from build123d import *

# Parameters (mm, degrees)
F0_W     = 120
F0_H     = 240
F0_R     = 2
F0_R_2   = 50.25
F1_DEPTH = 15
F0_R_3   = 1.75
F2_DEPTH = 12
F0_R_4   = 2.5
F0_R_5   = 51.75
F3_DEPTH = 10.5


with BuildPart() as f1:
    # F0 (on Right) → F1 (new body)
    with BuildSketch(Plane.YZ):
        with Locations((0, -1.592548)):
            Rectangle(F0_W, F0_H)
        with Locations((-49.999997, -113.592548)):
            Circle(F0_R, mode=Mode.SUBTRACT)
        with BuildLine():
            ThreePointArc((-43.965421, -1.013646), (0, 7.657452), (43.965421, -1.013646))
            ThreePointArc((43.965421, -1.013646), (46.58482, -2.757728), (48.328902, -5.377127))
            ThreePointArc((48.328902, -5.377127), (57, -49.342548), (48.328902, -93.307969))
            ThreePointArc((48.328902, -93.307969), (46.58482, -95.927368), (43.965421, -97.67145))
            ThreePointArc((43.965421, -97.67145), (0, -106.342548), (-43.965421, -97.67145))
            ThreePointArc((-43.965421, -97.67145), (-46.58482, -95.927368), (-48.328902, -93.307969))
            ThreePointArc((-48.328902, -93.307969), (-57, -49.342548), (-48.328902, -5.377127))
            ThreePointArc((-48.328902, -5.377127), (-46.58482, -2.757728), (-43.965421, -1.013646))
        make_face(mode=Mode.SUBTRACT)
        with Locations((50.000003, -113.592548)):
            Circle(F0_R, mode=Mode.SUBTRACT)
        with Locations((-49.999997, 110.407452)):
            Circle(F0_R, mode=Mode.SUBTRACT)
        with Locations((0.079908, 59.407452)):
            Circle(F0_R_2, mode=Mode.SUBTRACT)
        with Locations((50.000003, 110.407455)):
            Circle(F0_R, mode=Mode.SUBTRACT)
    extrude(amount=-F1_DEPTH)

    # F0 (on Right) → F2 (join)
    with BuildSketch(Plane.YZ):
        with Locations((0.079908, 59.407452)):
            Circle(F0_R_2)
        with Locations((-28.845534, 24.935452)):
            Circle(F0_R_3, mode=Mode.SUBTRACT)
        with Locations((-45.415495, 59.40745)):
            Circle(F0_R_3, mode=Mode.SUBTRACT)
        with Locations((-28.845534, 93.879452)):
            Circle(F0_R_3, mode=Mode.SUBTRACT)
        with Locations((29.005351, 24.935452)):
            Circle(F0_R_3, mode=Mode.SUBTRACT)
        with BuildLine():
            Line((-18.920092, 98.407452), (19.079908, 98.407452))
            ThreePointArc((19.079908, 98.407452), (21.201229, 97.528772), (22.079908, 95.407452))
            Line((22.079908, 95.407452), (22.079908, 23.407452))
            ThreePointArc((22.079908, 23.407452), (21.201229, 21.286132), (19.079908, 20.407452))
            Line((19.079908, 20.407452), (-18.920092, 20.407452))
            ThreePointArc((-18.920092, 20.407452), (-21.041412, 21.286132), (-21.920092, 23.407452))
            Line((-21.920092, 23.407452), (-21.920092, 95.407452))
            ThreePointArc((-21.920092, 95.407452), (-21.041412, 97.528772), (-18.920092, 98.407452))
        make_face(mode=Mode.SUBTRACT)
        with Locations((29.005351, 93.879452)):
            Circle(F0_R_3, mode=Mode.SUBTRACT)
        with Locations((45.292415, 59.40745)):
            Circle(F0_R_3, mode=Mode.SUBTRACT)
    extrude(amount=-F2_DEPTH)

    # F0 (on Right) → F3 (join)
    with BuildSketch(Plane.YZ):
        with BuildLine():
            ThreePointArc((48.328902, -5.377127), (46.58482, -2.757728), (43.965421, -1.013646))
            ThreePointArc((43.965421, -1.013646), (0, 7.657452), (-43.965421, -1.013646))
            ThreePointArc((-43.965421, -1.013646), (-46.58482, -2.757728), (-48.328902, -5.377127))
            ThreePointArc((-48.328902, -5.377127), (-57, -49.342548), (-48.328902, -93.307969))
            ThreePointArc((-48.328902, -93.307969), (-46.58482, -95.927368), (-43.965421, -97.67145))
            ThreePointArc((-43.965421, -97.67145), (0, -106.342548), (43.965421, -97.67145))
            ThreePointArc((43.965421, -97.67145), (46.58482, -95.927368), (48.328902, -93.307969))
            ThreePointArc((48.328902, -93.307969), (57, -49.342548), (48.328902, -5.377127))
        make_face()
        with Locations((-40.305087, -89.647635)):
            Circle(F0_R_4, mode=Mode.SUBTRACT)
        with Locations((-40.305087, -9.037462)):
            Circle(F0_R_4, mode=Mode.SUBTRACT)
        with Locations((40.305087, -89.647635)):
            Circle(F0_R_4, mode=Mode.SUBTRACT)
        with Locations((0, -49.342548)):
            Circle(F0_R_5, mode=Mode.SUBTRACT)
        with Locations((40.305087, -9.037462)):
            Circle(F0_R_4, mode=Mode.SUBTRACT)
    extrude(amount=-F3_DEPTH)


solid = f1.part
The model under review builds one solid part; all positions refer to its coordinate system, in mm. A direction names the side the tool comes from. Give positions to 0.01 mm unless a question says otherwise; leave off trailing zeros. Order: outer loops, then holes, each group sorted by start corner. A loop starts at its lowest first (then second) coordinate and runs counter-clockwise, first axis right, second up. Notation, with made-up numbers: M -30,-34 L -6,-34 A25 ccw -6,-7 Z; hole C 34.5,72.25 d5. An arc over 180 degrees is marked long. Use one line per item in the form item = value. Start each with the question number.
Item 1: The part is to be moulded in two halves that separate along Y. For faces 1 (the flat face through (0, -28, 27)), 2 (the flat face through (-7, 60, -3)), 3 (the cylindrical face through (-5.18, -42.29, -91.17)), say which applies: pulls with the +Y half, pulls with the -Y half, needs draft (parallel to the pull), parting line crosses it, or undercut.
Item 2: We need section A-A on z = 85. Give the boundary of the cut face in (x, y).
Item 3: Insertion check: pin 1 Ø5.5 at (y, z) = (-28.85, 24.94) entering from -X. The pin has a flat end and moves straight along its axis. Give the tip position at first contact, or say it passes through.
Item 4: For faces 4 (the flat face through (-6, 0, 98.407)), 5 (the cylindrical face through (-12.72, -46.55, -95.96)), 6 (the flat face through (-15, 9, 8)), list the 3-axis set-ups (+Z, -Z, +X, -X, +Y, -Y) from which the entire face can be reached by the end or side of a thin tool; tool diameter is ignored.
Item 5: We need section B-B on x = -6.75. Give the number of separate pieces and of enclosed holes in the cut face, plus the area to 3 significant figures.
Item 6: To check wall thickness, follow line 1 along Y through (x, z) = (-8.5, 85); line 2 along Z through (x, y) = (-9, -3); line 3 along Z through (x, y) = (-13, -25.5). State the ranges of each line that lie inside material, in increasing order. Write a range as from..to.
Item 7: We need section D-D on z = 31. Give the boundary of the cut face in (x, y), plus the area to 3 significant figures.
Item 8: We need section C-C on y = 0. Give the boundary of the cut face in (x, z), plus the area to 3 significant figures.
Completed:
q1.face_1 = needs draft
q1.face_2 = pulls with the +Y half
q1.face_3 = undercut
q2.outline = M -15,-60 L 0,-60 L 0,-21.92 L -12,-21.92 L -12,-43.16 L -15,-43.16 Z; M -15,43.32 L -12,43.32 L -12,22.08 L 0,22.08 L 0,60 L -15,60 Z
q3.pin_1 = -12
q4.face_4 = +X, -X
q4.face_5 = -X
q4.face_6 = +Z, -Z, -X, +Y, -Y
q5.separate_pieces = 1
q5.enclosed_holes = 16
q5.area = 16,800 mm²
q6.line_1 = -60..-21.92, 22.08..60
q6.line_2 = -121.59..-101.01, 2.32..20.41, 98.41..118.41
q6.line_3 = -121.59..-103.5, 4.81..16.16, 102.66..118.41
q7.outline = M -15,-60 L 0,-60 L 0,-21.92 L -12,-21.92 L -12,-41.37 L -15,-41.37 Z; M -15,41.53 L -12,41.53 L -12,22.08 L 0,22.08 L 0,60 L -15,60 Z
q7.area = 1,020 mm²
q8.outline = M -15,-121.59 L 0,-121.59 L 0,-101.09 L -10.5,-101.09 L -10.5,-106.34 L -15,-106.34 Z; M -15,7.66 L -10.5,7.66 L -10.5,2.41 L 0,2.41 L 0,20.41 L -12,20.41 L -12,9.16 L -15,9.16 Z; M -15,109.66 L -12,109.66 L -12,98.41 L 0,98.41 L 0,118.41 L -15,118.41 Z
q8.area = 763 mm²
